from build123d import *

# Parameters (mm, degrees)
BOSS_EXTRUDE1_DEPTH       = 4.826
M3X0_5_TAPPED_HOLE2_D     = 2.5
M3X0_5_TAPPED_HOLE3_D     = 2.5
M3X0_5_TAPPED_HOLE3_DEPTH = 5
M3X0_5_TAPPED_HOLE3_TIP   = 0.751075774
FILLET1_R                 = 2.5
FILLET2_R                 = 4


with BuildPart() as part:
    # Sketch1 → Boss-Extrude1 (new body)
    with BuildSketch(Plane.XY):
        Polygon((0, 0), (0, 13.5), (10, 13.5), (10, 20), (25, 20), (25, 7.5), (35, 7.5), (35, 0), align=None)
    extrude(amount=BOSS_EXTRUDE1_DEPTH)

    # M3x0.5 Tapped Hole2 (through all)
    with Locations(Plane.XY.offset(4.826)):
        with Locations((13.97024649, 12.44)):
            Hole(M3X0_5_TAPPED_HOLE2_D / 2)

    # M3x0.5 Tapped Hole3
    with Locations(Plane(origin=(0, 0, 0), x_dir=(-1, 0, 0), z_dir=(0, -1, 0))):
        with Locations((-16.73, -2.413), (-28.73, -2.413)):
            Hole(M3X0_5_TAPPED_HOLE3_D / 2, depth=M3X0_5_TAPPED_HOLE3_DEPTH)
            with Locations((0, 0, -(M3X0_5_TAPPED_HOLE3_DEPTH + M3X0_5_TAPPED_HOLE3_TIP / 2))):  # 118° drill point
                Cone(0, M3X0_5_TAPPED_HOLE3_D / 2, M3X0_5_TAPPED_HOLE3_TIP, mode=Mode.SUBTRACT)

    # Fillet1
    fillet1_edges = [part.edges().sort_by_distance(p)[0] for p in [
        (10, 20, 2.413),
        (10, 13.5, 2.413),
    ]]
    fillet(fillet1_edges, radius=FILLET1_R)

    # Fillet2
    fillet2_edges = [part.edges().sort_by_distance(p)[0] for p in [
        (25, 20, 2.413),
        (25, 7.5, 2.413),
        (35, 7.5, 2.413),
        (0, 13.5, 2.413),
    ]]
    fillet(fillet2_edges, radius=FILLET2_R)


solid = part.part
Model file for the job. Use its own axes, mm. A direction names the side the tool comes from. Round coordinates to 2 decimals unless told otherwise and drop trailing zeros. Order: outer loops, then holes, each group sorted by start corner. A loop starts at its lowest first (then second) coordinate and runs counter-clockwise, first axis right, second up.
(1) Drill centre lines: line 1 (Z direction, x = 28.73, y = 1.5); line 2 (X direction, y = 3.75, z = 0.4); line 3 (X direction, y = 2.25, z = 3.15). Where is each one in solid material? Low to high.
(2) Band-saw the part on B-B (z = 0.6). List the corners of the cut face in (x, y).
(3) 3-axis set-ups, long thin cutter, end or side, ignore diameter. For faces 4 (the face through (25, 14, 2)), 5 (the face through (0, 5, 2)), 6 (the face through (10, 17, 2)), 7 (the face through (29.885, 2.535, 2.892)): which of +Z, -Z, +X, -X, +Y, -Y reach the whole face in a straight line?
(4) Pin check, flat tips, straight feed: pin 1 (1.5 mm diameter, centred on y = 18, z = 2.5, fed in from -X); pin 2 (2 mm diameter, centred on x = 13.97, y = 12.44, fed in from -Z); pin 3 (1.5 mm diameter, centred on x = 26.5, y = 6, fed in from -Z); pin 4 (1.6 mm diameter, centred on x = 29.5, z = 3.5, fed in from +Y). Stop position of each tip, or through.
(5) Band-saw the part on D-D (x = 24). List the corners of the cut face in (y, z), then the cut area to 3 significant figures.
(6) Band-saw the part on A-A (y = 12.44). List the corners of the cut face in (x, z).
(7) Pull direction X, two halves, no side cores. Call faces 1 (the face through (30, 7.5, 2)), 2 (the face through (17.885, 2.535, 2.892)), 3 (the face through (33.859, 6.297, 2.447)): released by +X, released by -X, zero draft, split by the parting line, or undercut.
(8) Band-saw the part on C-C (y = 3). List the corners of the cut face in (x, z).
Verdict:
1. line 1: z = 0 to 1.16, 3.66 to 4.83
1. line 2: x = 0 to 34.99
1. line 3: x = 0 to 15.72, 17.74 to 27.72, 29.74 to 35
2. outline: (0, 0) - (35, 0) - (35, 3.5) arc R4 ccw to (31, 7.5) - (29, 7.5) arc R4 cw to (25, 11.5) - (25, 16) arc R4 ccw to (21, 20) - (12.5, 20) arc R2.5 ccw to (10, 17.5) - (10, 16) arc R2.5 cw to (7.5, 13.5) - (4, 13.5) arc R4 ccw to (0, 9.5) - close; hole circle Ø2.5 at (13.97, 12.44)
3. face 4: +Z, -Z, +X, +Y
3. face 5: +Z, -Z, -X, +Y, -Y
3. face 6: +Z, -Z, -X, +Y
3. face 7: -Y
4. pin 1: stops at x = 10
4. pin 2: passes through
4. pin 3: stops at z = 0
4. pin 4: stops at y = 7.51
5. outline: (0, 0) - (18.65, 0) - (18.65, 4.83) - (0, 4.83) - close
5. area: 90.0 mm2
6. outline: (1.29, 0) - (12.72, 0) - (12.72, 4.83) - (1.29, 4.83) - close; (15.22, 0) - (25, 0) - (25, 4.83) - (15.22, 4.83) - close
7. face 1: zero draft
7. face 2: undercut
7. face 3: released by +X
8. outline: (0, 0) - (35, 0) - (35, 4.83) - (0, 4.83) - close; hole circle Ø2.5 at (16.73, 2.41); hole circle Ø2.5 at (28.73, 2.41)
